Autodesk Inventor part; units mm, degrees
ref_plane "作業平面1" through (45, 0, 0) normal (1, 0, 0) x (0, 1, 0)
ref_plane "作業平面2" through (-45, 0, 0) normal (1, 0, 0) x (0, 1, 0)
ref_plane "作業平面3" through (0, 45, 0) normal (0, 1, 0) x (-1, 0, 0)
sketch "スケッチ1" plane through (0, 0, 0) normal (0, 0, 1) x (1, 0, 0)
  circle A0 centre (0, 0) radius 45
  circle A1 centre (0, 0) radius 11.5
  dimension "d0" = 90
  dimension "d1" = 23
extrude "押し出し1" add sketch "スケッチ1" along normal blind 8
sketch "スケッチ2" plane through (0, 0, 8) normal (0, 0, 1) x (1, 0, 0)
  line L0 (0, 0) -> (0, 16) construction
  circle A0 centre (0, 16) radius 2
  circle A1 centre (-16, 0) radius 2
  circle A2 centre (0, -16) radius 2
  circle A3 centre (16, 0) radius 2
  dimension "d4" = 16
  dimension "d5" = 4
  dimension "d8" = 360
extrude "押し出し2" cut sketch "スケッチ2" against normal blind 8
ref_plane "作業平面1" through (45, 0, 0) normal (1, 0, 0) x (0, 1, 0)
sketch "スケッチ3" plane through (45, 0, 0) normal (1, 0, 0) x (0, 1, 0)
  line L0 (0, 0) -> (0, 4) construction
  circle A0 centre (0, 4) radius 1.5
  dimension "d13" = 4
  dimension "d14" = 3
extrude "押し出し3" cut sketch "スケッチ3" against normal blind 10
ref_plane "作業平面2" through (-45, 0, 0) normal (1, 0, 0) x (0, 1, 0)
sketch "スケッチ4" plane through (-45, 0, 0) normal (1, 0, 0) x (0, 1, 0)
  line L0 (0, 0) -> (0, 4) construction
  circle A0 centre (0, 4) radius 1.5
  dimension "d20" = 4
  dimension "d21" = 3
extrude "押し出し4" cut sketch "スケッチ4" along normal blind 10
ref_plane "作業平面3" through (0, 45, 0) normal (0, 1, 0) x (-1, 0, 0)
sketch "スケッチ5" plane through (0, 45, 0) normal (0, 1, 0) x (-1, 0, 0)
  line L0 (0, 0) -> (0, 4) construction
  circle A0 centre (0, 4) radius 1.5
  dimension "d25" = 4
  dimension "d26" = 3
extrude "押し出し5" cut sketch "スケッチ5" against normal blind 10
ref_plane "作業平面4" through (0, -45, 0) normal (0, 1, 0) x (-1, 0, 0)
sketch "スケッチ6" plane through (0, -45, 0) normal (0, 1, 0) x (-1, 0, 0)
  line L0 (0, 0) -> (0, 4) construction
  circle A0 centre (0, 4) radius 1.5
  dimension "d30" = 4
  dimension "d31" = 3
extrude "押し出し6" cut sketch "スケッチ6" along normal blind 10
thread "ねじ2"
thread "ねじ3"
thread "ねじ4"
thread "ねじ5"
thread "ねじ10"
thread "ねじ11"
thread "ねじ12"
thread "ねじ13"
properties part number "Bottom1"
The listing builds one solid part. Answer for the finished solid, in the listing's coordinates (mm). A direction names the side the tool comes from. Give positions to 0.01 mm unless a question says otherwise; leave off trailing zeros. Write each loop counter-clockwise with the first axis right and the second up, starting at its lowest first coordinate (ties: lowest second). Pieces come first, ordered by that corner, then holes. Notation, with made-up numbers: (37.25, 14) -> (77.25, 14) arc R33 cw to (77.25, 49) -> close; hole circle Ø11 at (30.5, 50.5). An arc over 180 degrees is marked (long way). Write item = value, one per line. Start each with the question number.
1) Determine the mould class of faces 4 (the face through (-35, 0, 4)), 5 (the face through (-17.6, -1.2, 4.1)), 6 (the face through (-40.07, -0.195, 2.513)) for opening direction X: +X half, -X half, draft (parallel to the pull), parting line (faces both ways), or undercut.
2) The part is cut by section D-D, the plane y = -16. Determine the outline of the cut face in (x, z).
3) Each of these flat-tipped pins is pushed along its axis until it touches: pin 1 (4 mm diameter, centred on x = 16.5, z = 1, fed in from +Y); pin 2 (1.5 mm diameter, centred on x = -1.5, z = 3.5, fed in from -Y); pin 3 (3 mm diameter, centred on x = 16, y = 0, fed in from +Z); pin 4 (2 mm diameter, centred on x = 35.5, z = 7, fed in from -Y). Where does it stop, or does it pass through?
4) The part is cut by section B-B, the plane x = -16.5. Determine the outline of the cut face in (y, z), and give its area (3 significant figures).
5) Which of the six approach directions +Z, -Z, +X, -X, +Y, -Y give full straight-line access (tool end or side, diameter ignored) to faces 1 (the face through (-0.806, 40.07, 5.265)), 2 (the face through (0, -35, 4)), 3 (the face through (40.07, 0.806, 5.265))?
6) Straight lines are drawn through the part: line 1 along Y through (x, z) = (0, 5.25); line 2 along Z through (x, y) = (37, 0); line 3 along Y through (x, z) = (-5.5, 6). For each, find the intervals that lie inside material, in ascending order.
7) The part is cut by section C-C, the plane z = 4. Determine the outline of the cut face in (x, y) (3 decimals), and give its area (3 significant figures).
8) The part is cut by section A-A, the plane y = 0. Determine the outline of the cut face in (x, z), and give its area (3 significant figures).
Solutions:
q1.face_4 = -X half
q1.face_5 = undercut
q1.face_6 = draft
q2.outline = (-42.06, 0) -> (-2, 0) -> (-2, 8) -> (-42.06, 8) -> close; (2, 0) -> (42.06, 0) -> (42.06, 8) -> (2, 8) -> close
q3.pin_1 = 42.6
q3.pin_2 = -44.99
q3.pin_3 = through
q3.pin_4 = -28.89
q4.outline = (-41.87, 0) -> (-1.94, 0) -> (-1.94, 8) -> (-41.87, 8) -> close; (1.94, 0) -> (41.87, 0) -> (41.87, 8) -> (1.94, 8) -> close
q4.area = 639 mm²
q5.face_1 = +Y
q5.face_2 = -Y
q5.face_3 = +X
q6.line_1 = -35 to -18, -14 to -11.5, 11.5 to 14, 18 to 35
q6.line_2 = 0 to 2.5, 5.5 to 8
q6.line_3 = -44.66 to -10.1, 10.1 to 44.66
q7.outline = (-44.975, -1.5) arc R45 ccw to (-1.5, -44.975) -> (-1.5, -35) -> (1.5, -35) -> (1.5, -44.975) arc R45 ccw to (44.975, -1.5) -> (35, -1.5) -> (35, 1.5) -> (44.975, 1.5) arc R45 ccw to (1.5, 44.975) -> (1.5, 35) -> (-1.5, 35) -> (-1.5, 44.975) arc R45 ccw to (-44.975, 1.5) -> (-35, 1.5) -> (-35, -1.5) -> close; hole circle Ø4 at (-16, 0); hole circle Ø23 at (0, 0); hole circle Ø4 at (0, -16); hole circle Ø4 at (0, 16); hole circle Ø4 at (16, 0)
q7.area = 5,780 mm²
q8.outline = (-45, 0) -> (-18, 0) -> (-18, 8) -> (-45, 8) -> (-45, 5.5) -> (-35, 5.5) -> (-35, 2.5) -> (-45, 2.5) -> close; (-14, 0) -> (-11.5, 0) -> (-11.5, 8) -> (-14, 8) -> close; (11.5, 0) -> (14, 0) -> (14, 8) -> (11.5, 8) -> close; (18, 0) -> (45, 0) -> (45, 2.5) -> (35, 2.5) -> (35, 5.5) -> (45, 5.5) -> (45, 8) -> (18, 8) -> close
q8.area = 412 mm²
